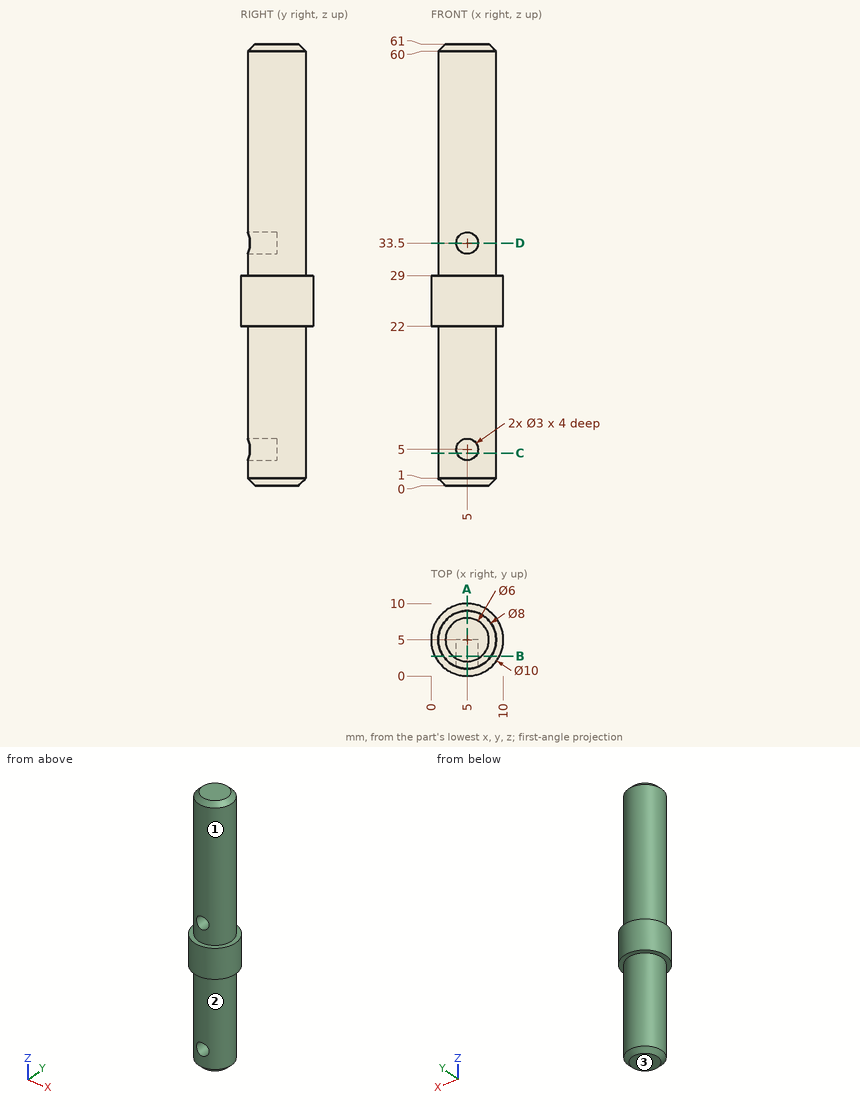
Input: dimensioned drawing with shaded views. Units: mm. Origin: part minimum x, y, z. A direction names the side the tool comes from. Coordinates: 2 decimals unless noted, no trailing zeros. Loops run counter-clockwise (first coordinate to the right, second up) from the corner with the lowest first, then second, coordinate; pieces in that order, holes last. Notation, with made-up numbers: M 59.5,39 L 79.5,39 A19 ccw 79.5,51 Z; hole C 18.5,-19 d10. An arc over 180 degrees is marked long. Use a Markdown table: item, result. Add a question column.
1) Set-up query: the marked faces 1, 2 and 3. Return all of +Z, -Z, +X, -X, +Y, -Y with unobstructed straight access to the full face (end or side cutting, diameter ignored); none if empty.
2) Section A-A, the plane x = 5. Return the cut outline in (y, z), plus the area to 3 significant figures.
3) Line query: L1, parallel to Z at x = 5, y = 3.35; L2, parallel to Z at x = 5, y = 1.9; L3, parallel to X at y = 3.45, z = 33.5. Output: solid intervals per line, ascending. Write a range as from..to.
4) Pin query (flat end, axial travel): P1, Ø0.9, axis at x = 4.5, z = 33, coming from the -Y side; P2, Ø2, axis at x = 4, z = 18, coming from the -Y side; P3, Ø3, axis at y = 2, z = 7, coming from the +X side; P4, Ø5, axis at y = 5.5, z = 29, coming from the +X side. Return the tip coordinate at first contact, or that it passes through.
5) Section D-D, the plane z = 33.5. Return the cut outline in (x, y).
6) Section B-B, the plane y = 2.75. Give the number of separate pieces and of enclosed holes in the cut face, plus the area to 3 significant figures.
7) Section C-C, the plane z = 4.5. Return the cut outline in (x, y), plus the area to 3 significant figures.
Answer below:
| question | item | result |
|---|---|---|
| 1 | face 1 | +Z |
| 1 | face 2 | -Z |
| 1 | face 3 | -Z, +X, -X, +Y, -Y |
| 2 | outline | M 0,22 L 1,22 L 1,6.5 L 5,6.5 L 5,3.5 L 1,3.5 L 1,1 L 2,0 L 8,0 L 9,1 L 9,22 L 10,22 L 10,29 L 9,29 L 9,60 L 8,61 L 2,61 L 1,60 L 1,35 L 5,35 L 5,32 L 1,32 L 1,29 L 0,29 Z |
| 2 | area | 476 mm2 |
| 3 | L1 | 0..3.5, 6.5..32, 35..61 |
| 3 | L2 | 0.1..3.5, 6.5..32, 35..60.9 |
| 3 | L3 | 1.31..3.5, 6.5..8.69 |
| 4 | P1 | y = 5 |
| 4 | P2 | y = 1 |
| 4 | P3 | x = 8.71 |
| 4 | P4 | x = 10 |
| 5 | outline | M 3.5,1.29 L 3.5,5 L 6.5,5 L 6.5,1.29 A4 ccw long Z |
| 6 | separate pieces | 1 |
| 6 | enclosed holes | 2 |
| 6 | area | 403 mm2 |
| 7 | outline | M 3.59,1.26 L 3.59,5 L 6.41,5 L 6.41,1.26 A4 ccw long Z |
| 7 | area | 39.2 mm2 |
